Solid Edge part; units mm, degrees
sketch "Sketch1" plane through (0, 0, 0) normal (0, 0, 1) x (1, 0, 0)
  circle A0 centre (0, 0) radius 42.5
  circle A1 centre (0, 0) radius 35
extrude "Protrusion1" add sketch "Sketch1" along normal blind 1.5
sketch "Sketch2" plane through (0, 0, 1.5) normal (0, 0, 1) x (1, 0, 0)
  line L0 (-33.5139, 12.0859) -> (-39.3095, 13.6388)
  line L1 (-39.3095, 13.6388) -> (-40.8624, 7.8432)
  line L2 (-40.8624, 7.8432) -> (-35.0668, 6.2903)
  line L3 (-35.0668, 6.2903) -> (-33.5139, 12.0859)
  line L4 (-37.4401, 18.1519) -> (-32.2439, 15.1519)
  line L5 (-32.2439, 15.1519) -> (-29.2439, 20.3481)
  line L6 (-29.2439, 20.3481) -> (-34.4401, 23.3481)
  line L7 (-34.4401, 23.3481) -> (-37.4401, 18.1519)
  line L8 (-27.2236, 22.981) -> (-22.981, 27.2236)
  line L9 (-22.981, 27.2236) -> (-27.2236, 31.4663)
  line L10 (-27.2236, 31.4663) -> (-31.4663, 27.2236)
  line L11 (-31.4663, 27.2236) -> (-27.2236, 22.981)
  line L12 (-23.3481, 34.4401) -> (-20.3481, 29.2439)
  line L13 (-20.3481, 29.2439) -> (-15.1519, 32.2439)
  line L14 (-15.1519, 32.2439) -> (-18.1519, 37.4401)
  line L15 (-18.1519, 37.4401) -> (-23.3481, 34.4401)
  line L16 (-12.0859, 33.5139) -> (-6.2903, 35.0668)
  line L17 (-6.2903, 35.0668) -> (-7.8432, 40.8624)
  line L18 (-7.8432, 40.8624) -> (-13.6388, 39.3095)
  line L19 (-13.6388, 39.3095) -> (-12.0859, 33.5139)
  line L20 (-3, 41.5) -> (-3, 35.5)
  line L21 (-3, 35.5) -> (3, 35.5)
  line L22 (3, 35.5) -> (3, 41.5)
  line L23 (3, 41.5) -> (-3, 41.5)
  line L24 (7.8432, 40.8624) -> (6.2903, 35.0668)
  line L25 (6.2903, 35.0668) -> (12.0859, 33.5139)
  line L26 (12.0859, 33.5139) -> (13.6388, 39.3095)
  line L27 (13.6388, 39.3095) -> (7.8432, 40.8624)
  line L28 (15.1519, 32.2439) -> (20.3481, 29.2439)
  line L29 (20.3481, 29.2439) -> (23.3481, 34.4401)
  line L30 (23.3481, 34.4401) -> (18.1519, 37.4401)
  line L31 (18.1519, 37.4401) -> (15.1519, 32.2439)
  line L32 (27.2236, 31.4663) -> (22.981, 27.2236)
  line L33 (22.981, 27.2236) -> (27.2236, 22.981)
  line L34 (27.2236, 22.981) -> (31.4663, 27.2236)
  line L35 (31.4663, 27.2236) -> (27.2236, 31.4663)
  line L36 (29.2439, 20.3481) -> (32.2439, 15.1519)
  line L37 (32.2439, 15.1519) -> (37.4401, 18.1519)
  line L38 (37.4401, 18.1519) -> (34.4401, 23.3481)
  line L39 (34.4401, 23.3481) -> (29.2439, 20.3481)
  line L40 (39.3095, 13.6388) -> (33.5139, 12.0859)
  line L41 (33.5139, 12.0859) -> (35.0668, 6.2903)
  line L42 (35.0668, 6.2903) -> (40.8624, 7.8432)
  line L43 (40.8624, 7.8432) -> (39.3095, 13.6388)
  line L44 (41.5, 3) -> (35.5, 3)
  line L45 (35.5, 3) -> (35.5, -3)
  line L46 (35.5, -3) -> (41.5, -3)
  line L47 (41.5, -3) -> (41.5, 3)
  line L48 (40.8624, -7.8432) -> (35.0668, -6.2903)
  line L49 (35.0668, -6.2903) -> (33.5139, -12.0859)
  line L50 (33.5139, -12.0859) -> (39.3095, -13.6388)
  line L51 (39.3095, -13.6388) -> (40.8624, -7.8432)
  line L52 (37.4401, -18.1519) -> (32.2439, -15.1519)
  line L53 (32.2439, -15.1519) -> (29.2439, -20.3481)
  line L54 (29.2439, -20.3481) -> (34.4401, -23.3481)
  line L55 (34.4401, -23.3481) -> (37.4401, -18.1519)
  line L56 (31.4663, -27.2236) -> (27.2236, -22.981)
  line L57 (27.2236, -22.981) -> (22.981, -27.2236)
  line L58 (22.981, -27.2236) -> (27.2236, -31.4663)
  line L59 (27.2236, -31.4663) -> (31.4663, -27.2236)
  line L60 (23.3481, -34.4401) -> (20.3481, -29.2439)
  line L61 (20.3481, -29.2439) -> (15.1519, -32.2439)
  line L62 (15.1519, -32.2439) -> (18.1519, -37.4401)
  line L63 (18.1519, -37.4401) -> (23.3481, -34.4401)
  line L64 (13.6388, -39.3095) -> (12.0859, -33.5139)
  line L65 (12.0859, -33.5139) -> (6.2903, -35.0668)
  line L66 (6.2903, -35.0668) -> (7.8432, -40.8624)
  line L67 (7.8432, -40.8624) -> (13.6388, -39.3095)
  line L68 (3, -41.5) -> (3, -35.5)
  line L69 (3, -35.5) -> (-3, -35.5)
  line L70 (-3, -35.5) -> (-3, -41.5)
  line L71 (-3, -41.5) -> (3, -41.5)
  line L72 (-7.8432, -40.8624) -> (-6.2903, -35.0668)
  line L73 (-6.2903, -35.0668) -> (-12.0859, -33.5139)
  line L74 (-12.0859, -33.5139) -> (-13.6388, -39.3095)
  line L75 (-13.6388, -39.3095) -> (-7.8432, -40.8624)
  line L76 (-18.1519, -37.4401) -> (-15.1519, -32.2439)
  line L77 (-15.1519, -32.2439) -> (-20.3481, -29.2439)
  line L78 (-20.3481, -29.2439) -> (-23.3481, -34.4401)
  line L79 (-23.3481, -34.4401) -> (-18.1519, -37.4401)
  line L80 (-27.2236, -31.4663) -> (-22.981, -27.2236)
  line L81 (-22.981, -27.2236) -> (-27.2236, -22.981)
  line L82 (-27.2236, -22.981) -> (-31.4663, -27.2236)
  line L83 (-31.4663, -27.2236) -> (-27.2236, -31.4663)
  line L84 (-34.4401, -23.3481) -> (-29.2439, -20.3481)
  line L85 (-29.2439, -20.3481) -> (-32.2439, -15.1519)
  line L86 (-32.2439, -15.1519) -> (-37.4401, -18.1519)
  line L87 (-37.4401, -18.1519) -> (-34.4401, -23.3481)
  line L88 (-39.3095, -13.6388) -> (-33.5139, -12.0859)
  line L89 (-33.5139, -12.0859) -> (-35.0668, -6.2903)
  line L90 (-35.0668, -6.2903) -> (-40.8624, -7.8432)
  line L91 (-40.8624, -7.8432) -> (-39.3095, -13.6388)
  line L92 (-41.5, -3) -> (-35.5, -3)
  line L93 (-35.5, -3) -> (-35.5, 3)
  line L94 (-35.5, 3) -> (-41.5, 3)
  line L95 (-41.5, 3) -> (-41.5, -3)
extrude "ExtrudedCutout_2" cut sketch "Sketch2" against normal blind 0.5
properties material "ABS Plastic, medium impact"
Verification items for the finished model (mm, model axes). Coordinates: 2 decimals unless noted, no trailing zeros. Write each loop counter-clockwise with the first axis right and the second up, starting at its lowest first coordinate (ties: lowest second). Pieces come first, ordered by that corner, then holes. Notation, with made-up numbers: (-30, 18.5) - (-4, 18.5) arc R22 cw to (-4, 40.5) - close; hole circle Ø6 at (74.5, 43). An arc over 180 degrees is marked (long way). Answer as a JSON object with one key per item and string values.
(1) Thickness scan on line 1 along Y through (x, z) = (0, 1.25); line 2 along Y through (x, z) = (0, 0.4); line 3 along X through (y, z) = (-1, 0.4). Record the ranges inside material, lowest first.
Report:
{"line 1": "-42.5 to -41.5, -35.5 to -35, 35 to 35.5, 41.5 to 42.5", "line 2": "-42.5 to -35, 35 to 42.5", "line 3": "-42.49 to -34.99, 34.99 to 42.49"}
(2) Gauge pin test, flat end, axial feed: pin 1 Ø4 at (x, y) = (-33, 18.5) entering from +Z. Record the tip position at first contact, or that the pin passes through.
Report:
{"pin 1": "z = 1"}
(3) Cross-section at C-C on z = 0.5. Record the cut outline in (x, y), plus the area to 3 significant figures.
Report:
{"outline": "circle Ø85 at (0, 0); hole circle Ø70 at (0, 0)", "area": "1,830 mm^2"}
(4) Cross-section at A-A on x = 0. Record the cut outline in (y, z).
Report:
{"outline": "(-42.5, 0) - (-35, 0) - (-35, 1.5) - (-35.5, 1.5) - (-35.5, 1) - (-41.5, 1) - (-41.5, 1.5) - (-42.5, 1.5) - close; (35, 0) - (42.5, 0) - (42.5, 1.5) - (41.5, 1.5) - (41.5, 1) - (35.5, 1) - (35.5, 1.5) - (35, 1.5) - close"}
